Geometry: final body of the model. Coordinates: model frame, mm. Face numbers are marked on the shaded views. A direction names the side the tool comes from. Give positions to 0.01 mm unless a question says otherwise; leave off trailing zeros. Write each loop counter-clockwise with the first axis right and the second up, starting at its lowest first coordinate (ties: lowest second). Pieces come first, ordered by that corner, then holes. Notation, with made-up numbers: (-32, 27.25) - (-28, 27.25) arc R12 ccw to (-28, 39.25) - close; hole circle Ø4 at (-14, 26.5). An arc over 180 degrees is marked (long way). One line per question, with ' | ' between items. Start each with the question number.
```python
from build123d import *

# Parameters (mm, degrees)
SKETCH1_W           = 30
SKETCH1_H           = 29
BOSS_EXTRUDE1_DEPTH = 8
SKETCH2_W           = 24
SKETCH2_H           = 8
CUT_EXTRUDE1_DEPTH  = 8
CUT_EXTRUDE2_DEPTH  = 8
CUT_EXTRUDE3_DEPTH  = 6
BELT_CUTOUT_W       = 9
BELT_CUTOUT_H       = 5
CUT_EXTRUDE4_DEPTH  = 30


with BuildPart() as part:
    # Sketch1 → Boss-Extrude1 (new body)
    with BuildSketch(Plane(origin=(0, 0, 0), x_dir=(1, 0, 0), z_dir=(0, 1, 0))):
        with Locations((-14.236607143, -13.569196429)):
            Rectangle(SKETCH1_W, SKETCH1_H)
    extrude(amount=BOSS_EXTRUDE1_DEPTH)

    # Sketch2 → Cut-Extrude1 (cut)
    with BuildSketch(Plane(origin=(0, 8, 0), x_dir=(1, 0, 0), z_dir=(0, 1, 0))):
        with Locations((-14.236607143, -6.069196429)):
            Rectangle(SKETCH2_W, SKETCH2_H)
        with Locations((-14.236607143, -17.069196429)):
            Rectangle(SKETCH2_W, SKETCH2_H)
    extrude(amount=-CUT_EXTRUDE1_DEPTH, mode=Mode.SUBTRACT)

    # Sketch3 → Cut-Extrude2 (cut)
    with BuildSketch(Plane(origin=(0, 8, 0), x_dir=(1, 0, 0), z_dir=(0, 1, 0))):
        Polygon((-29.236607143, -22.519140749), (-22.236607143, -28.069196429), (-29.236607143, -28.069196429), align=None)
    extrude(amount=-CUT_EXTRUDE2_DEPTH, mode=Mode.SUBTRACT)

    # cutout → Cut-Extrude3 (cut)
    with BuildSketch(Plane.XZ):
        Polygon((-0.736607143, 0.569196429), (-27.736607143, 0.569196429), (-27.736607143, 21.794168589), (-21.714109927, 26.569196429), (-0.736607143, 26.569196429), align=None)
    extrude(amount=-CUT_EXTRUDE3_DEPTH, mode=Mode.SUBTRACT)

    # belt_cutout → Cut-Extrude4 (cut)
    with BuildSketch(Plane.ZY.offset(29.236607143)):
        with Locations((11.069196429, 2.5)):
            Rectangle(BELT_CUTOUT_W, BELT_CUTOUT_H)
    extrude(amount=-CUT_EXTRUDE4_DEPTH, mode=Mode.SUBTRACT)


solid = part.part
```
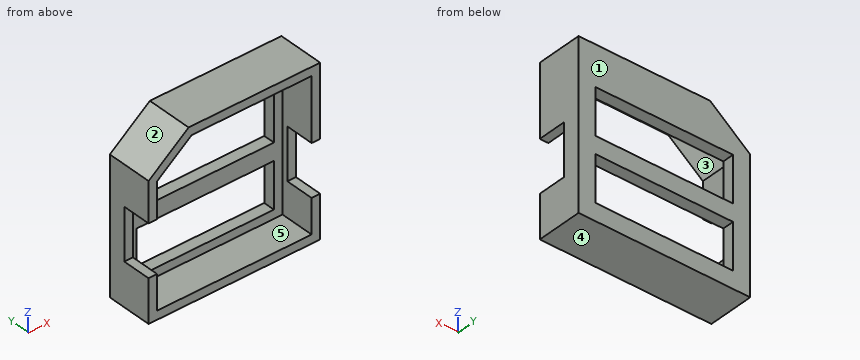
1) Pull-direction query (X, two-part tool) for the marked faces 1, 2 and 3; classes: +X half, -X half, draft (parallel to the pull), parting line (faces both ways), or undercut.
2) Section C-C, the plane z = 17.75. Output: boundary loops of the cut face in (x, y), plus the area to 3 significant figures.
3) Section B-B, the plane y = 1.5. Output: boundary loops of the cut face in (x, z), plus the area to 3 significant figures.
4) First-contact query: pin 1 Ø2 at (x, z) = (-8.5, 9.5) entering from +Y; pin 2 Ø8 at (x, z) = (-21, 17) entering from -Y; pin 3 Ø1.6 at (x, y) = (-28.5, 3) entering from +Z. Flat tips, straight axial feed; report the tip coordinate or a pass-through.
5) Reachability of the marked faces 4 and 5 from +Z, -Z, +X, -X, +Y, -Y: full face, straight path, thin tool, end or side. Return the list, or none.
6) Line query: L1, parallel to Z at x = -9, y = 7.5; L2, parallel to X at y = 4.5, z = 1; L3, parallel to Z at x = -17.75, y = 4. Output: solid intervals per line, ascending.
7) Section A-A, the plane x = -7. Output: boundary loops of the cut face in (y, z), plus the area to 3 significant figures.
8) Section D-D, the plane y = 7. Output: boundary loops of the cut face in (x, z), plus the area to 3 significant figures.
Answer key:
1) face 1: draft | face 2: -X half | face 3: undercut
2) outline: (-29.24, 0) - (-27.74, 0) - (-27.74, 6) - (-26.24, 6) - (-26.24, 8) - (-29.24, 8) - close; (-2.24, 6) - (-0.74, 6) - (-0.74, 0) - (0.76, 0) - (0.76, 8) - (-2.24, 8) - close | area: 30.0 mm^2
3) outline: (-29.24, -0.93) - (0.76, -0.93) - (0.76, 6.57) - (-0.74, 6.57) - (-0.74, 0.57) - (-27.74, 0.57) - (-27.74, 6.57) - (-29.24, 6.57) - close; (-29.24, 15.57) - (-27.74, 15.57) - (-27.74, 21.79) - (-21.71, 26.57) - (-0.74, 26.57) - (-0.74, 15.57) - (0.76, 15.57) - (0.76, 28.07) - (-22.24, 28.07) - (-29.24, 22.52) - close | area: 136 mm^2
4) pin 1: y = 8 | pin 2: y = 6 | pin 3: z = 23.74
5) face 4: -Z, +X, -X, +Y, -Y | face 5: -Y
6) L1: -0.93 to 2.07, 10.07 to 13.07, 21.07 to 28.07 | L2: -29.24 to -27.74, -0.74 to 0.76 | L3: -0.93 to 0.57, 26.57 to 28.07
7) outline: (0, -0.93) - (8, -0.93) - (8, 2.07) - (6, 2.07) - (6, 0.57) - (0, 0.57) - close; (0, 26.57) - (6, 26.57) - (6, 21.07) - (8, 21.07) - (8, 28.07) - (0, 28.07) - close; (6, 10.07) - (8, 10.07) - (8, 13.07) - (6, 13.07) - close | area: 44.0 mm^2
8) outline: (-29.24, -0.93) - (0.76, -0.93) - (0.76, 28.07) - (-22.24, 28.07) - (-29.24, 22.52) - close; hole (-26.24, 2.07) - (-2.24, 2.07) - (-2.24, 10.07) - (-26.24, 10.07) - close; hole (-26.24, 13.07) - (-2.24, 13.07) - (-2.24, 21.07) - (-26.24, 21.07) - close | area: 467 mm^2
